from build123d import *


with BuildPart() as part:
    # Sketch1 → Revolve1 (revolve)
    with BuildSketch(Plane.XY):
        with BuildLine():
            Line((-85.973820479, 0), (-85.973820479, 3.9497))
            Line((-85.973820479, 3.9497), (37.698779521, 3.9497))
            ThreePointArc((37.698779521, 3.9497), (39.589789562, 3.135625716), (41.629711619, 2.8575))
            Line((41.629711619, 2.8575), (48.163579521, 2.8575))
            Line((48.163579521, 2.8575), (48.163579521, 2.3495))
            Line((48.163579521, 2.3495), (49.142936851, 2.3495))
            Line((49.142936851, 2.3495), (54.984769387, 1.145946184))
            Line((54.984769387, 1.145946184), (54.984769387, 0.914360397))
            Line((54.984769387, 0.914360397), (58.679179521, 0))
            Line((58.679179521, 0), (-85.973820479, 0))
        make_face()
    revolve(axis=Axis((-85.973820479, 0, 0), (1, 0, 0)))


solid = part.part
Work out the finished part from the listing and answer in its coordinate system (mm). A direction names the side the tool comes from. Give positions to 0.01 mm unless a question says otherwise; leave off trailing zeros. Loops run counter-clockwise (first coordinate to the right, second up) from the corner with the lowest first, then second, coordinate; pieces in that order, holes last. Notation, with made-up numbers: (73.5, 25.25) -> (130.5, 25.25) arc R22 ccw to (130.5, 61.25) -> close; hole circle Ø9 at (-21.5, 24.5). An arc over 180 degrees is marked (long way). Use a Markdown table: item, result. Add a question column.
1. Flat-ended cylindrical pins translate along their axes: pin 1 Ø1 at (x, z) = (-49.5, 2.5) entering from +Y; pin 2 Ø1.5 at (x, z) = (16.5, 1.5) entering from +Y; pin 3 Ø1 at (x, y) = (-55.5, -1) entering from -Z. Find the tip coordinate at first contact, or state that the pin passes through.
2. For faces 1 (the flat face through (-85.974, 0, 0)), 2 (the cylindrical face through (48.66, -0.31, 2.33)), determine the directions among +Z, -Z, +X, -X, +Y, -Y from which every point of the face is accessible in a straight line to the end or side of a thin tool.
3. Section A-A on x = 1.5 is taken. Determine the outline of the cut face in (y, z), and give its area (3 significant figures).
4. Find the intervals of material crossed by probe 1 along Y at (x, z) = (-4.5, -2.75); probe 2 along Y at (x, z) = (-49, -0.25); probe 3 along X at (y, z) = (2.25, 1), in increasing order.
Results below:
| question | item | result |
|---|---|---|
| 1 | pin 1 | stops at y = 3.41 |
| 1 | pin 2 | stops at y = 3.88 |
| 1 | pin 3 | stops at z = -3.92 |
| 2 | face 1 | +Z, -Z, -X, +Y, -Y |
| 2 | face 2 | +X |
| 3 | outline | circle Ø7.9 at (0, 0) |
| 3 | area | 49.0 mm^2 |
| 4 | probe 1 | y = -2.84 to 2.84 |
| 4 | probe 2 | y = -3.94 to 3.94 |
| 4 | probe 3 | x = -85.97 to 48.16 |
